```python
from build123d import *

# Parameters (mm, degrees)
F0_W     = 148
F0_H     = 100
F1_DEPTH = 8
F2_SIZE  = 3
F3_W     = 69
F3_H     = 24
F3_W_2   = 33
F3_H_2   = 20
F4_DEPTH = 6.6
F5_SIZE  = 1


with BuildPart() as f1:
    # F0 (on Top) → F1 (new body)
    with BuildSketch(Plane.XY):
        Rectangle(F0_W, F0_H)
    extrude(amount=F1_DEPTH)

    # F2
    f2_edges = [f1.edges().sort_by_distance(p)[0] for p in [
        (-74, -50, 4),
        (-74, 50, 4),
        (74, 50, 4),
        (74, -50, 4),
    ]]
    chamfer(f2_edges, length=F2_SIZE)

    # F3 (on face) → F4 (cut)
    with BuildSketch(Plane.XY.offset(8)):
        with Locations((-36, 34.5)):
            Rectangle(F3_W, F3_H)
        with Locations((36, 34.5)):
            Rectangle(F3_W, F3_H)
        with Locations((-54, 9.5)):
            Rectangle(F3_W_2, F3_H_2)
        with Locations((-18, 9.5)):
            Rectangle(F3_W_2, F3_H_2)
        with Locations((18, 9.5)):
            Rectangle(F3_W_2, F3_H_2)
        with Locations((54, 9.5)):
            Rectangle(F3_W_2, F3_H_2)
        with Locations((54, -13.5)):
            Rectangle(F3_W_2, F3_H_2)
        with Locations((18, -13.5)):
            Rectangle(F3_W_2, F3_H_2)
        with Locations((-18, -13.5)):
            Rectangle(F3_W_2, F3_H_2)
        with Locations((-54, -13.5)):
            Rectangle(F3_W_2, F3_H_2)
        with Locations((-54, -36.5)):
            Rectangle(F3_W_2, F3_H_2)
        with Locations((-18, -36.5)):
            Rectangle(F3_W_2, F3_H_2)
        with Locations((18, -36.5)):
            Rectangle(F3_W_2, F3_H_2)
        with Locations((54, -36.5)):
            Rectangle(F3_W_2, F3_H_2)
    extrude(amount=-F4_DEPTH, mode=Mode.SUBTRACT)

    # F5
    f5_edges = [f1.edges().sort_by_distance(p)[0] for p in [
        (70.5, 46.5, 4.7),
        (-70.5, 46.5, 4.7),
        (70.5, -46.5, 4.7),
        (-70.5, -46.5, 4.7),
    ]]
    chamfer(f5_edges, length=F5_SIZE)


solid = f1.part
```
CAD build for the part. Positions are in the model's coordinates, mm. Give positions to 0.01 mm unless a question says otherwise; leave off trailing zeros. Write each loop counter-clockwise with the first axis right and the second up, starting at its lowest first coordinate (ties: lowest second). Pieces come first, ordered by that corner, then holes. Notation, with made-up numbers: (20, 12.25) -> (37, 12.25) arc R14 cw to (37, 36.25) -> close; hole circle Ø5 at (71.5, 38.25). An arc over 180 degrees is marked (long way). Write each question's results on one line, items separated by ' | '.
1. Cut at B-B, the plane x = 39.5. Write the cut outline in (y, z), then the cut area to 3 significant figures.
Geometry check:
outline: (-50, 0) -> (50, 0) -> (50, 8) -> (46.5, 8) -> (46.5, 1.4) -> (22.5, 1.4) -> (22.5, 8) -> (19.5, 8) -> (19.5, 1.4) -> (-0.5, 1.4) -> (-0.5, 8) -> (-3.5, 8) -> (-3.5, 1.4) -> (-23.5, 1.4) -> (-23.5, 8) -> (-26.5, 8) -> (-26.5, 1.4) -> (-46.5, 1.4) -> (-46.5, 8) -> (-50, 8) -> close | area: 246 mm²
2. Wall check: probe 1 along X at (y, z) = (2.5, 5.5); probe 2 along Y at (x, z) = (13.5, 6.5); probe 3 along X at (y, z) = (44, 2.5). Give the ranges that are in metal, low to high. Write a range as [from, to].
Geometry check:
probe 1: [-74, -70.5], [-37.5, -34.5], [-1.5, 1.5], [34.5, 37.5], [70.5, 74] | probe 2: [-50, -46.5], [-26.5, -23.5], [-3.5, -0.5], [19.5, 22.5], [46.5, 50] | probe 3: [-74, -70.5], [-1.5, 1.5], [70.5, 74]
3. Cut at D-D, the plane y = 12.5. Write the cut outline in (x, z), then the cut area to 3 significant figures.
Geometry check:
outline: (-74, 0) -> (74, 0) -> (74, 8) -> (70.5, 8) -> (70.5, 1.4) -> (37.5, 1.4) -> (37.5, 8) -> (34.5, 8) -> (34.5, 1.4) -> (1.5, 1.4) -> (1.5, 8) -> (-1.5, 8) -> (-1.5, 1.4) -> (-34.5, 1.4) -> (-34.5, 8) -> (-37.5, 8) -> (-37.5, 1.4) -> (-70.5, 1.4) -> (-70.5, 8) -> (-74, 8) -> close | area: 313 mm²
4. Drop a flat-ended pin along its axis: P1, Ø10, axis at x = -20.5, y = 28, coming from the +Z side. Give the stop position or say it passes through.
Geometry check:
P1: z = 1.4
5. Cut at A-A, the plane y = 39. Write the cut outline in (x, z), then the cut area to 3 significant figures.
Geometry check:
outline: (-74, 0) -> (74, 0) -> (74, 8) -> (70.5, 8) -> (70.5, 1.4) -> (1.5, 1.4) -> (1.5, 8) -> (-1.5, 8) -> (-1.5, 1.4) -> (-70.5, 1.4) -> (-70.5, 8) -> (-74, 8) -> close | area: 273 mm²
6. Cut at C-C, the plane z = 4.25. Give the number of separate pieces and of enclosed holes in the cut face, then the cut area to 3 significant figures.
Geometry check:
separate pieces: 1 | enclosed holes: 14 | area: 3,550 mm²
7. Two-plate mould, pull along Y, no slides. Class faces 1 (the flat face through (73, -48, 4)), 2 (the flat face through (-18, -36, 1.4)): pulls with the +Y half, pulls with the -Y half, needs draft (parallel to the pull), parting line crosses it, or undercut.
Geometry check:
face 1: pulls with the -Y half | face 2: undercut
